Part model, mm, in its own coordinate system. Face numbers are marked on the shaded views. A direction names the side the tool comes from. Give positions to 0.01 mm unless a question says otherwise; leave off trailing zeros. Order: outer loops, then holes, each group sorted by start corner. A loop starts at its lowest first (then second) coordinate and runs counter-clockwise, first axis right, second up. Notation, with made-up numbers: M 24,-12 L 46,-12 A16 ccw 46,13 Z; hole C 21,-4 d11. An arc over 180 degrees is marked long. Answer as a JSON object with one key per item and string values.
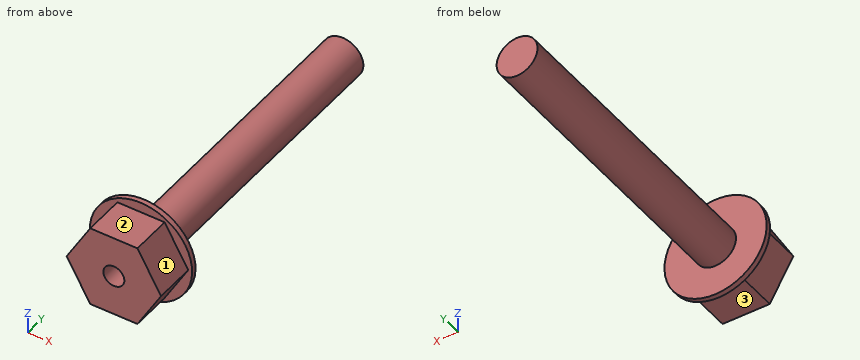
from build123d import *

# Parameters (mm, degrees)
SKETCH1_R           = 3.175
BOSS_EXTRUDE1_DEPTH = 46.355
SKETCH3_R           = 7.9375
BOSS_EXTRUDE3_DEPTH = 0.79375
BOSS_EXTRUDE4_DEPTH = 6.35


# Read off the part's stored shape, not the designer's step: AdvancedHole1
with BuildPart() as part:
    # Sketch1 → Boss-Extrude1 (new body)
    with BuildSketch(Plane(origin=(0, 0, 0), x_dir=(1, 0, 0), z_dir=(0, 1, 0))):
        with Locations(Location((0, 0, 0), (0, 0, 90))):
            Circle(SKETCH1_R)
    extrude(amount=BOSS_EXTRUDE1_DEPTH)

    # Sketch3 → Boss-Extrude3 (add)
    with BuildSketch(Plane.XZ):
        with Locations(Location((0, 0, 0), (0, 0, 270))):
            Circle(SKETCH3_R)
    extrude(amount=BOSS_EXTRUDE3_DEPTH)

    # Sketch4 → Boss-Extrude4 (add)
    with BuildSketch(Plane.XZ.offset(0.79375)):
        Polygon((3.666174209, 6.35), (-3.666174209, 6.35), (-7.332348419, 0), (-3.666174209, -6.35), (3.666174209, -6.35), (7.332348419, 0), align=None)
    extrude(amount=BOSS_EXTRUDE4_DEPTH)

    # AdvancedHole1 outline → AdvancedHole1 (revolve, cut)
    with BuildSketch(Plane.XY):
        Polygon((1.63195, -7.14375), (1.63195, 3.96875), (0, 4.949324487), (0, -7.14375), align=None)
    revolve(axis=Axis((0, 0, 0), (0, 1, 0)), mode=Mode.SUBTRACT)


solid = part.part
1. Cut at A-A on z = 5.5. Give the cut face in (x, y), plus the area to 3 significant figures.
Worked answers:
{"outline": "M -5.72,-0.79 L -4.16,-0.79 L -4.16,-7.14 L 4.16,-7.14 L 4.16,-0.79 L 5.72,-0.79 L 5.72,0 L -5.72,0 Z", "area": "61.9 mm^2"}
2. Which spindle directions (+Z, -Z, +X, -X, +Y, -Y) get a long thin tool onto all of the face, cutting with end or side? Do the marked faces 1, 2 and 3. Say none if no direction does.
Worked answers:
{"face 1": "+Z, +X, -Y", "face 2": "+Z, +X, -X, -Y", "face 3": "-Z, +X, -X, -Y"}
3. Pin check, flat tips, straight feed: P1, Ø5, axis at x = -1.5, y = 19, coming from the -Z side (3 decimals); P2, Ø2.5, axis at x = 0, z = 0, coming from the -Y side; P3, Ø1, axis at y = 25, z = -0.5, coming from the -X side (3 decimals). Stop position of each tip, or through.
Worked answers:
{"P1": "stops at z = -3.175", "P2": "stops at y = 4.2", "P3": "stops at x = -3.175"}
4. Probe line 1 along X through (y, z) = (1.25, 0) (3 decimals); line 2 along Z through (x, y) = (0, -2.25); line 3 along X through (y, z) = (-1.5, 0). List the from-to ranges inside material, lowest first.
Worked answers:
{"line 1": "x = -3.175 to -1.632, 1.632 to 3.175", "line 2": "z = -6.35 to -1.63, 1.63 to 6.35", "line 3": "x = -7.33 to -1.63, 1.63 to 7.33"}
5. Cut at B-B on y = 15. Give the cut face in (x, z) (3 decimals).
Worked answers:
{"outline": "C 0,0 d6.35"}
6. Cut at C-C on z = -4. Give the cut face in (x, y), plus the area to 3 significant figures.
Worked answers:
{"outline": "M -6.86,-0.79 L -5.02,-0.79 L -5.02,-7.14 L 5.02,-7.14 L 5.02,-0.79 L 6.86,-0.79 L 6.86,0 L -6.86,0 Z", "area": "74.7 mm^2"}
